For this review, take the finished solid that the model builds, in its own axes (mm). A direction names the side the tool comes from. Coordinates: 2 decimals unless noted, no trailing zeros. Loops run counter-clockwise (first coordinate to the right, second up) from the corner with the lowest first, then second, coordinate; pieces in that order, holes last. Notation, with made-up numbers: (52.25, -24.75) -> (109.25, -24.75) arc R24 ccw to (109.25, -11.75) -> close; hole circle Ø2 at (-2.5, -30). An arc over 180 degrees is marked (long way). Answer in a Markdown table with one row per item.
from build123d import *

# Parameters (mm, degrees)
F0_W     = 1066.8
F0_H     = 457.2
F1_DEPTH = 19.05
F2_W     = 19.05
F2_H     = 438.15
F3_DEPTH = 425.45
F4_DEPTH = 196.85
F6_W     = 19.05
F6_H     = 215.9
F7_DEPTH = 82.55


with BuildPart() as f1:
    # F0 (on Top) → F1 (new body)
    with BuildSketch(Plane.XY):
        Rectangle(F0_W, F0_H)
    extrude(amount=F1_DEPTH)

    # F2 (on face) → F3 (join)
    with BuildSketch(Plane.XY.offset(19.05)):
        with Locations((523.875, 9.525)):
            Rectangle(F2_W, F2_H)
        with Locations((-523.875, 9.525)):
            Rectangle(F2_W, F2_H)
    extrude(amount=F3_DEPTH)

    # F2 (on face) → F4 (join)
    with BuildSketch(Plane.XY.offset(19.05)):
        Polygon((-514.35, -209.55), (-533.4, -209.55), (-533.4, -228.6), (533.4, -228.6), (533.4, -209.55), (514.35, -209.55), align=None)
    extrude(amount=F4_DEPTH)

    # F6 (on face) → F7 (join)
    with BuildSketch(Plane.XZ.offset(228.6)):
        with Locations((-523.875, 107.95)):
            Rectangle(F6_W, F6_H)
        with Locations((523.875, 107.95)):
            Rectangle(F6_W, F6_H)
    extrude(amount=F7_DEPTH)


solid = f1.part
Item 1: For L1, parallel to X at y = -31.5, z = 299; L2, parallel to Z at x = -61, y = 83; L3, parallel to Y at x = 26, z = 114, list the stretches that pass through material, from the lowest coordinate up.
Worked answers:
| item | result |
|---|---|
| L1 | -533.4 to -514.35, 514.35 to 533.4 |
| L2 | 0 to 19.05 |
| L3 | -228.6 to -209.55 |
Item 2: Take a section at A-A, the plane z = 227.5. State the section outline as (x, y) points, and give its area (3 significant figures).
Worked answers:
| item | result |
|---|---|
| outline | (-533.4, -209.55) -> (-514.35, -209.55) -> (-514.35, 228.6) -> (-533.4, 228.6) -> close; (514.35, -209.55) -> (533.4, -209.55) -> (533.4, 228.6) -> (514.35, 228.6) -> close |
| area | 16,700 mm² |
Item 3: Take a section at B-B, the plane y = -127. State the section outline as (x, z) points, and give its area (3 significant figures).
Worked answers:
| item | result |
|---|---|
| outline | (-533.4, 0) -> (533.4, 0) -> (533.4, 444.5) -> (514.35, 444.5) -> (514.35, 19.05) -> (-514.35, 19.05) -> (-514.35, 444.5) -> (-533.4, 444.5) -> close |
| area | 36,500 mm² |
Item 4: Insertion check: pin 1 (1.5 mm diameter, centred on x = 90.5, z = 58, fed in from +Y); pin 2 (8 mm diameter, centred on x = -238, z = 75, fed in from -Y); pin 3 (9.5 mm diameter, centred on x = -526, z = 289.5, fed in from -Y). Each pin has a flat end and moves straight along its axis. Give the tip position at first contact, or say it passes through.
Worked answers:
| item | result |
|---|---|
| pin 1 | y = -209.55 |
| pin 2 | y = -228.6 |
| pin 3 | y = -209.55 |
Item 5: For faces 1 (the flat face through (-514.35, 6, 229)), 2 (the flat face through (-533.4, -37, 219)), 3 (the flat face through (-82, -226, 215.9)), 4 (the flat face through (-7, 22, 0)), 5 (the flat face through (514.35, -269, 106)), list the 3-axis set-ups (+Z, -Z, +X, -X, +Y, -Y) from which the entire face can be reached by the end or side of a thin tool; tool diameter is ignored.
Worked answers:
| item | result |
|---|---|
| face 1 | +Z, +Y |
| face 2 | +Z, -Z, -X, +Y, -Y |
| face 3 | +Z, +X, -X, -Y |
| face 4 | -Z, +X, -X, +Y, -Y |
| face 5 | +Z, -Z, -Y |
Item 6: Take a section at C-C, the plane x = 304. State the section outline as (y, z) points.
Worked answers:
| item | result |
|---|---|
| outline | (-228.6, 0) -> (228.6, 0) -> (228.6, 19.05) -> (-209.55, 19.05) -> (-209.55, 215.9) -> (-228.6, 215.9) -> close |
Item 7: Take a section at D-D, the plane z = 114. State the section outline as (x, y) points.
Worked answers:
| item | result |
|---|---|
| outline | (-533.4, -311.15) -> (-514.35, -311.15) -> (-514.35, -228.6) -> (514.35, -228.6) -> (514.35, -311.15) -> (533.4, -311.15) -> (533.4, 228.6) -> (514.35, 228.6) -> (514.35, -209.55) -> (-514.35, -209.55) -> (-514.35, 228.6) -> (-533.4, 228.6) -> close |
